from build123d import *

# Parameters (mm, degrees)
SKETCH_1_R      = 0.75
SKETCH_1_R_2    = 4.25
EXTRUDE_1_DEPTH = 2
SKETCH_1_3_R    = 3
SKETCH_1_3_R_2  = 1.5
EXTRUDE_2_DEPTH = 1
SKETCH_1_4_R    = 4.25
SKETCH_1_4_R_2  = 3
EXTRUDE_3_DEPTH = 5.5


with BuildPart() as part:
    # Sketch 1 → Extrude 1 (new body)
    with BuildSketch(Plane(origin=(0, 0, 0), x_dir=(1, 0, 0), z_dir=(0, 1, 0))):
        with BuildLine():
            Line((-5.297526475, 5.297526475), (-16.85, 2.939387691))
            ThreePointArc((-16.85, 2.939387691), (-19.25, 0), (-16.85, -2.939387691))
            Line((-16.85, -2.939387691), (-5.297526475, -5.297526475))
            Line((-5.297526475, -5.297526475), (-2.939387691, -16.85))
            ThreePointArc((-2.939387691, -16.85), (0, -19.25), (2.939387691, -16.85))
            Line((2.939387691, -16.85), (5.297526475, -5.297526475))
            Line((5.297526475, -5.297526475), (16.85, -2.939387691))
            ThreePointArc((16.85, -2.939387691), (19.25, 0), (16.85, 2.939387691))
            Line((16.85, 2.939387691), (5.297526475, 5.297526475))
            Line((5.297526475, 5.297526475), (2.939387691, 16.85))
            ThreePointArc((2.939387691, 16.85), (0, 19.25), (-2.939387691, 16.85))
            Line((-2.939387691, 16.85), (-5.297526475, 5.297526475))
        make_face()
        with Locations(Location((13.333333333, 0, 0), (0, 0, 270))):
            Circle(SKETCH_1_R, mode=Mode.SUBTRACT)
        with Locations(Location((0, -16.25, 0), (0, 0, 270))):
            Circle(SKETCH_1_R, mode=Mode.SUBTRACT)
        with Locations(Location((0, -13.333333333, 0), (0, 0, 270))):
            Circle(SKETCH_1_R, mode=Mode.SUBTRACT)
        with Locations(Location((0, -10.416666667, 0), (0, 0, 270))):
            Circle(SKETCH_1_R, mode=Mode.SUBTRACT)
        with Locations(Location((0, -7.5, 0), (0, 0, 270))):
            Circle(SKETCH_1_R, mode=Mode.SUBTRACT)
        with Locations(Location((-16.25, 0, 0), (0, 0, 270))):
            Circle(SKETCH_1_R, mode=Mode.SUBTRACT)
        with BuildLine():
            ThreePointArc((-12.583333333, 0), (-13.333333333, -0.75), (-14.083333333, 0))
            ThreePointArc((-14.083333333, 0), (-13.333333333, 0.75), (-12.583333333, 0))
        make_face(mode=Mode.SUBTRACT)
        with BuildLine():
            ThreePointArc((-9.666666667, 0), (-10.416666667, -0.75), (-11.166666667, 0))
            ThreePointArc((-11.166666667, 0), (-10.416666667, 0.75), (-9.666666667, 0))
        make_face(mode=Mode.SUBTRACT)
        with Locations(Location((-7.5, 0, 0), (0, 0, 270))):
            Circle(SKETCH_1_R, mode=Mode.SUBTRACT)
        with Locations(Location((0, 0, 0), (0, 0, 270))):
            Circle(SKETCH_1_R_2, mode=Mode.SUBTRACT)
        with Locations(Location((0, 7.5, 0), (0, 0, 270))):
            Circle(SKETCH_1_R, mode=Mode.SUBTRACT)
        with Locations(Location((7.5, 0, 0), (0, 0, 270))):
            Circle(SKETCH_1_R, mode=Mode.SUBTRACT)
        with Locations(Location((10.416666667, 0, 0), (0, 0, 270))):
            Circle(SKETCH_1_R, mode=Mode.SUBTRACT)
        with BuildLine():
            ThreePointArc((0, 11.166666667), (0.75, 10.416666667), (0, 9.666666667))
            ThreePointArc((0, 9.666666667), (-0.75, 10.416666667), (0, 11.166666667))
        make_face(mode=Mode.SUBTRACT)
        with BuildLine():
            ThreePointArc((0, 14.083333333), (0.75, 13.333333333), (0, 12.583333333))
            ThreePointArc((0, 12.583333333), (-0.75, 13.333333333), (0, 14.083333333))
        make_face(mode=Mode.SUBTRACT)
        with Locations(Location((0, 16.25, 0), (0, 0, 270))):
            Circle(SKETCH_1_R, mode=Mode.SUBTRACT)
        with Locations(Location((16.25, 0, 0), (0, 0, 270))):
            Circle(SKETCH_1_R, mode=Mode.SUBTRACT)
    extrude(amount=EXTRUDE_1_DEPTH)



with BuildPart() as body_2:
    # Sketch 1_3 → Extrude 2 (new body)
    with BuildSketch(Plane(origin=(0, 0, 0), x_dir=(1, 0, 0), z_dir=(0, 1, 0))):
        with Locations(Location((0, 0, 0), (0, 0, 270))):
            Circle(SKETCH_1_3_R)
        with Locations(Location((0, 0, 0), (0, 0, 270))):
            Circle(SKETCH_1_3_R_2, mode=Mode.SUBTRACT)
    extrude(amount=EXTRUDE_2_DEPTH)


with BuildPart() as part_1:
    add(part.part)

    add(body_2.part)  # Extrude 3 merges body 2
    # Sketch 1_4 → Extrude 3 (add)
    with BuildSketch(Plane(origin=(0, 0, 0), x_dir=(1, 0, 0), z_dir=(0, 1, 0))):
        with Locations(Location((0, 0, 0), (0, 0, 270))):
            Circle(SKETCH_1_4_R)
        with Locations(Location((0, 0, 0), (0, 0, 270))):
            Circle(SKETCH_1_4_R_2, mode=Mode.SUBTRACT)
    extrude(amount=EXTRUDE_3_DEPTH)


solid = part_1.part
Read the model definition and answer for the solid it produces. Units are mm, in the model's axes. A direction names the side the tool comes from. Give positions to 0.01 mm unless a question says otherwise; leave off trailing zeros. Loops run counter-clockwise (first coordinate to the right, second up) from the corner with the lowest first, then second, coordinate; pieces in that order, holes last. Notation, with made-up numbers: (11, 39.5) -> (29, 39.5) arc R10 cw to (29, 55.5) -> close; hole circle Ø9 at (26, 13.25). An arc over 180 degrees is marked (long way). Answer as CSV lines item,"result".
Item 1: Find section A-A on z = 7.5. Give the vertices of the cut face in (x, y), plus the area to 3 significant figures.
Returned:
outline,"(-4.85, 0) -> (-0.75, 0) -> (-0.75, 2) -> (-4.85, 2) -> close; (0.75, 0) -> (4.85, 0) -> (4.85, 2) -> (0.75, 2) -> close"
area,"16.4 mm²"
Item 2: Each of these flat-tipped pins is pushed along its axis until it touches: pin 1 (2 mm diameter, centred on x = 0, z = -13.33, fed in from +Y); pin 2 (1.5 mm diameter, centred on y = 1.5, z = -11.5, fed in from +X); pin 3 (1.5 mm diameter, centred on y = 4, z = -15, fed in from +X); pin 4 (1.5 mm diameter, centred on x = 1, y = 3.5, fed in from +Z). Where does it stop, or does it pass through?
Returned:
pin 1,"stops at y = 2"
pin 2,"stops at x = 4.18"
pin 3,"passes through"
pin 4,"stops at z = 4.24"
Item 3: Find section B-B on x = -16.25. Give the vertices of the cut face in (y, z), plus the area to 3 significant figures.
Returned:
outline,"(0, -3.06) -> (2, -3.06) -> (2, -0.75) -> (0, -0.75) -> close; (0, 0.75) -> (2, 0.75) -> (2, 3.06) -> (0, 3.06) -> close"
area,"9.25 mm²"
Item 4: Find section C-C on x = 0. State how many separate pieces and enclosed holes the cut face has, plus the area to 4 significant figures.
Returned:
separate pieces,"10"
enclosed holes,"0"
area,"52.75 mm²"
Item 5: For faces 1 (the face through (0.9, 3.22, 2.86)), 2 (the face through (-4.102, 0.986, -11.155)), determine the directions among +Z, -Z, +X, -X, +Y, -Y from which every point of the face is accessible in a straight line to the end or side of a thin tool.
Returned:
face 1,"+Y"
face 2,"-Z, -X, +Y, -Y"
Item 6: Consider line 1 (Y direction, x = -2.5, z = 12.5); line 2 (Z direction, x = 13.5, y = 0.8); line 3 (Z direction, x = 10, y = 1.75). Determine where each line is inside the solid, lowest interval first. Write a range as [from, to].
Returned:
line 1,"y = [0, 2]"
line 2,"z = [-3.62, -0.73], [0.73, 3.62]"
line 3,"z = [-4.34, -0.62], [0.62, 4.34]"
Item 7: Determine the mould class of faces 3 (the face through (11.155, 0.986, -4.102)), 4 (the face through (-17, 1, 0)), 5 (the face through (0.225, 0.986, 14.049)), 6 (the face through (4.102, 0.986, 11.155)) for opening direction Z: +Z half, -Z half, draft (parallel to the pull), parting line (faces both ways), or undercut.
Returned:
face 3,"-Z half"
face 4,"undercut"
face 5,"undercut"
face 6,"+Z half"
